Verification items for the finished model (mm, model axes). Face numbers are marked on the shaded views. Round coordinates to 2 decimals unless told otherwise and drop trailing zeros. Order: outer loops, then holes, each group sorted by start corner. A loop starts at its lowest first (then second) coordinate and runs counter-clockwise, first axis right, second up. Notation, with made-up numbers: (69, 79) -> (93, 79) arc R15 ccw to (93, 87) -> close; hole circle Ø10 at (34, 64). An arc over 180 degrees is marked (long way). Return JSON: item names as keys, results as strings. Group by question number.
1) Section check A-A on x = -38. Enter the section's corners in (y, z), plus the area to 3 significant figures.
2) Section check D-D on y = 27.5. Enter the section's corners in (x, z), plus the area to 3 significant figures.
3) Scan lines: L1, parallel to Y at x = -61.5, z = 10.25; L2, parallel to X at y = 22, z = 0.5; L3, parallel to X at y = 40.5, z = 1. Record each from-to range of solid material in increasing order.
4) Depth check by flat-ended pin: pin 1 (4.5 mm diameter, centred on y = 62.5, z = 3.5, fed in from +X); pin 2 (2 mm diameter, centred on x = -35.5, z = 0.5, fed in from -Y). Enter the tip coordinate at first touch or a pass-through.
5) Draft check along Y on the marked faces 1, 2 and 3. Enter one of: pulls with the +Y half, pulls with the -Y half, needs draft (parallel to the pull), parting line crosses it, or undercut.
6) Section check C-C on y = 5. Enter the section's corners in (x, z), plus the area to 3 significant figures.
7) Section check B-B on z = 3.5. Enter the section's corners in (x, y), plus the area to 3 significant figures.
```python
from build123d import *

# Parameters (mm, degrees)
F0_W      = 134
F0_H      = 69
F1_DEPTH  = 2
F2_W      = 81
F2_H      = 2
F3_DEPTH  = 4
F4_W      = 81
F4_H      = 4
F5_DEPTH  = 3
F6_DEPTH  = 7
F7_DEPTH  = 3
F8_W      = 81
F8_H      = 1
F9_DEPTH  = 0.5
F10_DEPTH = 1
F11_W     = 13
F11_H     = 2
F12_DEPTH = 4
F13_W     = 13
F13_H     = 4
F14_DEPTH = 10
F15_DEPTH = 3
F16_W     = 13
F16_H     = 0.9976745471
F17_DEPTH = 0.5
F18_W     = 81
F18_H     = 2
F19_DEPTH = 4
F20_W     = 81
F20_H     = 4
F21_DEPTH = 10
F22_DEPTH = 3
F23_W     = 81
F23_H     = 1
F24_DEPTH = 0.5
F25_W     = 26
F25_H     = 2
F26_DEPTH = 4
F27_W     = 26
F27_H     = 4
F28_DEPTH = 10
F29_DEPTH = 3
F30_W     = 26
F30_H     = 1
F31_DEPTH = 0.5
F33_DEPTH = 2.001
F34_W     = 15
F34_H     = 44
F35_DEPTH = 12.001
F36_W     = 7
F36_H     = 19
F36_W_2   = 15
F36_W_3   = 12
F37_DEPTH = 12.001
F40_DEPTH = 12.001


with BuildPart() as f1:
    # F0 (on Top) → F1 (new body)
    with BuildSketch(Plane.XY):
        with Locations((-4.8879205883, 25.1932881936)):
            Rectangle(F0_W, F0_H)
    extrude(amount=F1_DEPTH)

    # F2 (on face) → F3 (join)
    with BuildSketch(Plane.XZ.offset(9.3067118064)):
        with Locations((16.6120794117, 1)):
            Rectangle(F2_W, F2_H)
    extrude(amount=F3_DEPTH)

    # F4 (on face) → F5 (join)
    with BuildSketch(Plane.XY.offset(2)):
        with Locations((16.6120794117, -11.3067118064)):
            Rectangle(F4_W, F4_H)
    extrude(amount=F5_DEPTH)

    # F6 (add): a face of the model
    f6_faces = [f1.faces().sort_by_distance(p)[0] for p in [
        (16.6120794117, -11.3067118064, 5),
    ]]
    extrude(f6_faces, amount=F6_DEPTH)

    # F7 (cut): a face of the model
    f7_faces = [f1.faces().sort_by_distance(p)[0] for p in [
        (16.6120794117, -9.3067118064, 7),
    ]]
    extrude(f7_faces, amount=-F7_DEPTH, mode=Mode.SUBTRACT)

    # F8 (on face) → F9 (join)
    with BuildSketch(Plane(origin=(0, -12.3067118064, 0), x_dir=(-1, 0, 0), z_dir=(0, 1, 0))):
        with Locations((-16.6120794117, 11.5)):
            Rectangle(F8_W, F8_H)
    extrude(amount=F9_DEPTH)

    # F10 (cut): a face of the model
    f10_faces = [f1.faces().sort_by_distance(p)[0] for p in [
        (-23.8879205883, -11.3067118064, 0.1264911064),
    ]]
    extrude(f10_faces, amount=-F10_DEPTH, mode=Mode.SUBTRACT)

    # F11 (on face) → F12 (join)
    with BuildSketch(Plane.XZ.offset(9.3067118064)):
        with Locations((-60.3879205883, 1)):
            Rectangle(F11_W, F11_H)
    extrude(amount=F12_DEPTH)

    # F13 (on face) → F14 (join)
    with BuildSketch(Plane.XY.offset(2)):
        with Locations((-60.3879205883, -11.3067118064)):
            Rectangle(F13_W, F13_H)
    extrude(amount=F14_DEPTH)

    # F15 (cut): a face of the model
    f15_faces = [f1.faces().sort_by_distance(p)[0] for p in [
        (-60.3879205883, -9.3067118064, 7),
    ]]
    extrude(f15_faces, amount=-F15_DEPTH, mode=Mode.SUBTRACT)

    # F16 (on face) → F17 (join)
    with BuildSketch(Plane(origin=(0, -12.3067118064, 0), x_dir=(-1, 0, 0), z_dir=(0, 1, 0))):
        with Locations((60.3879205883, 11.5011627264)):
            Rectangle(F16_W, F16_H)
    extrude(amount=F17_DEPTH)

    # F18 (on face) → F19 (join)
    with BuildSketch(Plane(origin=(0, 59.6932881936, 0), x_dir=(-1, 0, 0), z_dir=(0, 1, 0))):
        with Locations((-16.6120794117, 1)):
            Rectangle(F18_W, F18_H)
    extrude(amount=F19_DEPTH)

    # F20 (on face) → F21 (join)
    with BuildSketch(Plane.XY.offset(2)):
        with Locations((16.6120794117, 61.6932881936)):
            Rectangle(F20_W, F20_H)
    extrude(amount=F21_DEPTH)

    # F22 (cut): a face of the model
    f22_faces = [f1.faces().sort_by_distance(p)[0] for p in [
        (16.6120794117, 59.6932881936, 7),
    ]]
    extrude(f22_faces, amount=-F22_DEPTH, mode=Mode.SUBTRACT)

    # F23 (on face) → F24 (join)
    with BuildSketch(Plane.XZ.offset(-62.6932881936)):
        with Locations((16.6120794117, 11.5)):
            Rectangle(F23_W, F23_H)
    extrude(amount=F24_DEPTH)

    # F25 (on face) → F26 (join)
    with BuildSketch(Plane(origin=(0, 59.6932881936, 0), x_dir=(-1, 0, 0), z_dir=(0, 1, 0))):
        with Locations((53.8879205883, 1)):
            Rectangle(F25_W, F25_H)
    extrude(amount=F26_DEPTH)

    # F27 (on face) → F28 (join)
    with BuildSketch(Plane.XY.offset(2)):
        with Locations((-53.8879205883, 61.6932881936)):
            Rectangle(F27_W, F27_H)
    extrude(amount=F28_DEPTH)

    # F29 (cut): a face of the model
    f29_faces = [f1.faces().sort_by_distance(p)[0] for p in [
        (-53.8879205883, 59.6932881936, 7),
    ]]
    extrude(f29_faces, amount=-F29_DEPTH, mode=Mode.SUBTRACT)

    # F30 (on face) → F31 (join)
    with BuildSketch(Plane.XZ.offset(-62.6932881936)):
        with Locations((-53.8879205883, 11.5)):
            Rectangle(F30_W, F30_H)
    extrude(amount=F31_DEPTH)

    # F32 (on face) → F33 (cut, through all)
    with BuildSketch(Plane.XY.offset(2)):
        Polygon((-71.8879205883, 52.6932881936), (-66.8879205883, 59.6932881936), (-71.8879205883, 59.6932881936), align=None)
        Polygon((-66.8879205883, -9.3067118064), (-71.8879205883, -2.3067118064), (-71.8879205883, -9.3067118064), align=None)
        Polygon((62.1120794117, -9.3067118064), (62.1120794117, -2.3067118064), (57.1120794117, -9.3067118064), align=None)
        Polygon((62.1120794117, 59.6932881936), (57.1120794117, 59.6932881936), (62.1120794117, 52.6932881936), align=None)
    extrude(amount=-F33_DEPTH, mode=Mode.SUBTRACT)

    # F34 (on face) → F35 (cut, through all)
    with BuildSketch(Plane(origin=(0, 0, 0), x_dir=(1, 0, 0), z_dir=(0, 0, -1))):
        with Locations((-48.3879205883, -24.6932881936)):
            Rectangle(F34_W, F34_H)
    extrude(amount=-F35_DEPTH, mode=Mode.SUBTRACT)

    # F36 (on face) → F37 (cut, through all)
    with BuildSketch(Plane(origin=(0, 0, 0), x_dir=(1, 0, 0), z_dir=(0, 0, -1))):
        with Locations((-59.3879205883, -24.1932881936)):
            Rectangle(F36_W, F36_H)
        with Locations((-48.3879205883, -24.1932881936)):
            Rectangle(F36_W_2, F36_H)
        with Locations((-34.8879205883, -24.1932881936)):
            Rectangle(F36_W_3, F36_H)
    extrude(amount=-F37_DEPTH, mode=Mode.SUBTRACT)

    # F39 (on face) → F40 (cut, through all)
    with BuildSketch(Plane(origin=(0, 0, 0), x_dir=(1, 0, 0), z_dir=(0, 0, -1))):
        Polygon((43.3054530231, -55.5370226502), (49.5563223958, -55.5370226502), (49.5563223958, -39.2849373539), (29.9500417569, -25.5961895548), (23.4002765373, -29.8256016073), (43.3054530231, -43.723033039), align=None)
        Polygon((23.4002765373, -29.8256016073), (29.9500417569, -25.5961895548), (23.2038749613, -20.8861388534), (16.6541097417, -25.1155509059), align=None)
        Polygon((23.2038749613, -20.8861388534), (29.9500417569, -25.5961895548), (49.5563223958, -12.9357296973), (49.5563223958, 5.9177065827), (43.3054530231, 5.9177065827), (43.3054530231, -7.9058481593), align=None)
        Polygon((16.6541097417, -25.1155509059), (23.2038749613, -20.8861388534), (-15.187051918, 5.9177065827), (-19.3186867982, 0), align=None)
        Polygon((-15.187051918, -54.7427866621), (23.4002765373, -29.8256016073), (16.6541097417, -25.1155509059), (-19.3186867982, -48.3444414305), align=None)
    extrude(amount=-F40_DEPTH, mode=Mode.SUBTRACT)


solid = f1.part
```
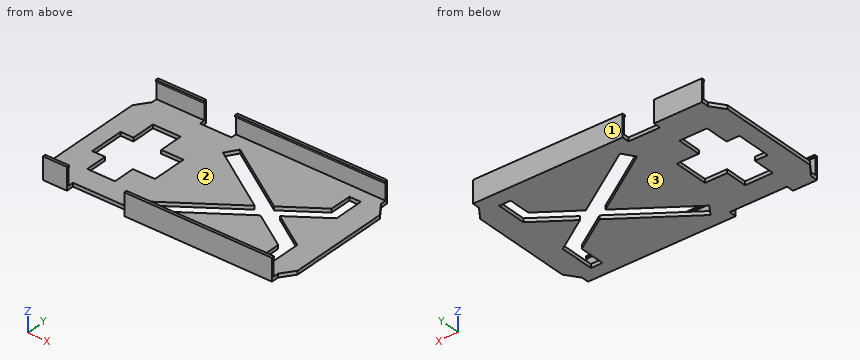
Check result:
{
 "1": {"outline": "(-9.31, 0) -> (14.69, 0) -> (14.69, 2) -> (-9.31, 2) -> close; (33.69, 0) -> (59.69, 0) -> (59.69, 2) -> (33.69, 2) -> close", "area": "100 mm^2"},
 "2": {"outline": "(-71.89, 0) -> (-62.89, 0) -> (-62.89, 2) -> (-71.89, 2) -> close; (-28.89, 0) -> (12.96, 0) -> (12.96, 2) -> (-28.89, 2) -> close; (32.68, 0) -> (62.11, 0) -> (62.11, 2) -> (32.68, 2) -> close", "area": "161 mm^2"},
 "3": {"L1": "-13.31 to -12.31, 62.69 to 63.69", "L2": "-71.89 to -62.89, -28.89 to 12.19, 35.52 to 62.11", "L3": "-71.89 to -55.89, -40.89 to -7.17, 6.87 to 38.69, 49.56 to 62.11"},
 "4": {"pin 1": "x = 57.11", "pin 2": "y = -9.31"},
 "5": {"face 1": "pulls with the +Y half", "face 2": "undercut", "face 3": "needs draft"},
 "6": {"outline": "(-71.89, 0) -> (-55.89, 0) -> (-55.89, 2) -> (-71.89, 2) -> close; (-40.89, 0) -> (-12.16, 0) -> (-12.16, 2) -> (-40.89, 2) -> close; (0.45, 0) -> (43.31, 0) -> (43.31, 2) -> (0.45, 2) -> close; (49.56, 0) -> (62.11, 0) -> (62.11, 2) -> (49.56, 2) -> close", "area": "200 mm^2"},
 "7": {"outline": "(-66.89, -13.31) -> (-53.89, -13.31) -> (-53.89, -12.31) -> (-66.89, -12.31) -> close; (-66.89, 62.69) -> (-40.89, 62.69) -> (-40.89, 63.69) -> (-66.89, 63.69) -> close; (-23.89, 62.69) -> (57.11, 62.69) -> (57.11, 63.69) -> (-23.89, 63.69) -> close; (-22.89, -13.31) -> (57.11, -13.31) -> (57.11, -12.31) -> (-22.89, -12.31) -> close", "area": "200 mm^2"}
}
